Can you work these out from the model? Positions are in its coordinate system, mm. A direction names the side the tool comes from. Give positions to 0.01 mm unless a question says otherwise; leave off trailing zeros. Loops run counter-clockwise (first coordinate to the right, second up) from the corner with the lowest first, then second, coordinate; pieces in that order, holes last. Notation, with made-up numbers: M 7.25,76 L 59.25,76 A18 ccw 59.25,97 Z; hole C -4,61.25 d4. An arc over 180 degrees is marked long. Answer as a JSON object with one key per item and string values.
Autodesk Inventor part; units mm, degrees
ref_plane "YZ Plane" through (0, 0, 0) normal (1, 0, 0) x (0, 1, 0)
ref_plane "XZ Plane" through (0, 0, 0) normal (0, 1, 0) x (-1, 0, 0)
ref_plane "XY Plane" through (0, 0, 0) normal (0, 0, 1) x (1, 0, 0)
sketch "Skizze1" plane through (0, 0, 0) normal (0, 0, 1) x (1, 0, 0)
  line L0 (0, -0.6) -> (0, 3.6)
  line L1 (-31.5, 0) -> (31.5, 0)
  line L2 (31.5, 0) -> (31.5, 3)
  line L3 (31.5, 3) -> (-31.5, 3)
  line L4 (-31.5, 3) -> (-31.5, 0)
  dimension "d2" = 63
  dimension "d3" = 3
revolve "Umdrehung1" add sketch "Skizze1" angle 360 about axis through (-31.5, 0, 0) along (1, 0, 0)
thread "Gewinde1"
chamfer "Fase1" distance 0.3 angle 45 1 edges at (31.5, -3, 0)
sketch "Skizze2" plane through (0, 0, 0) normal (0, 0, 1) x (1, 0, 0)
  line L0 (-31.5, -3) -> (-31.5, 3)
  line L1 (31.2, -3) -> (31.2, 3)
  line L2 (-58.1911, 0) -> (44.3485, 0)
  line L3 (0, -4.8487) -> (0, 8.0921)
  arc A0 (-34.9614, 3) -> (-43.9614, 0) centre (-38.9614, 0) ccw
  arc A1 (-34.9614, 3) -> (-31.5, 3) centre (-33.2307, 4.7589) ccw
  line L4 (-31.5, -3) -> (-31.5, 3)
  line L5 (-43.9614, 0) -> (-31.5, 0)
  line L6 (-31.5, 3) -> (-31.5, 0)
  point P0 (0, 0)
  dimension "d10" = 5
revolve "Umdrehung2" add sketch "Skizze2" angle 360 about axis through (-43.9614, 0, 0) along (1, 0, 0)
properties part number "M6x60" material "Stahl, hochfest, niedrig legiert"
1) For faces 1 (the cylindrical face through (-1, -3, 0)), 2 (the flat face through (31.5, 0, 0)), which set-ups out of +Z, -Z, +X, -X, +Y, -Y let a thin tool reach every point of the face, with its end or its side?
Answer list:
{"face 1": "+X", "face 2": "+Z, -Z, +X, +Y, -Y"}
2) Suppose I cut it at A-A, the plane y = 0. Write out the boundary of the cut face in (x, z), and give its area (3 significant figures).
Answer list:
{"outline": "M -34.96,-3 A2.47 cw -31.5,-3 L 31.2,-3 L 31.5,-2.7 L 31.5,2.7 L 31.2,3 L -31.5,3 A2.47 cw -34.96,3 A5 ccw long Z", "area": "470 mm^2"}
3) Suppose I cut it at C-C, the plane x = 6.5. Write out the boundary of the cut face in (y, z), and give its area (3 significant figures).
Answer list:
{"outline": "C 0,0 d6", "area": "28.3 mm^2"}
4) Suppose I cut it at D-D, the plane z = -4. Write out the boundary of the cut face in (x, y), and give its area (3 significant figures).
Answer list:
{"outline": "C -38.96,0 d6", "area": "28.3 mm^2"}
5) Will these pins go through, and if not, where does the flat tip stop? pin 1 Ø6 at (x, y) = (-36.5, -3.5) entering from +Z; pin 2 Ø2 at (x, z) = (-8.5, -1) entering from +Y; pin 3 Ø3 at (x, y) = (-10, 1.5) entering from +Z.
Answer list:
{"pin 1": "z = 4.83", "pin 2": "y = 3", "pin 3": "z = 3"}
6) Please list where these lines run through material, in increasing order: line 1 along Z through (x, y) = (4, 0); line 2 along X through (y, z) = (2.75, 1); line 3 along Z through (x, y) = (6.5, -1.5). Write a range as from..to.
Answer list:
{"line 1": "-3..3", "line 2": "-43.02..-34.88, -31.58..31.27", "line 3": "-2.6..2.6"}
